Read the model definition and answer for the solid it produces. Units are mm, in the model's axes. Round coordinates to 2 decimals unless told otherwise and drop trailing zeros. Use one line per item in the form item = value. Start each with the question number.
Autodesk Inventor part; units mm, degrees
ref_plane "YZ Plane" through (0, 0, 0) normal (1, 0, 0) x (0, 1, 0)
ref_plane "XZ Plane" through (0, 0, 0) normal (0, 1, 0) x (-1, 0, 0)
ref_plane "XY Plane" through (0, 0, 0) normal (0, 0, 1) x (1, 0, 0)
ref_plane "Work Plane1" through (-113.4922, 95.6302, 200.3599) normal (-0.0001, 0, -1) x (0, -1, 0)
sketch "Sketch1" plane through (-113.4922, 95.6302, 200.3599) normal (-0.0001, 0, -1) x (0, -1, 0)
  line L0 (212.1169, -104.14) -> (330.2269, -104.14)
  line L1 (117.2921, 3.175) -> (320.7139, 3.175)
  line L2 (320.7139, 3.175) -> (320.7139, -104.14)
  line L3 (320.7139, -104.14) -> (117.2921, -104.14)
  line L4 (117.2921, -104.14) -> (117.2921, 3.175)
  circle A0 centre (129.9921, -79.375) radius 2.667
  circle A1 centre (129.9921, -53.975) radius 2.667
  circle A2 centre (129.9921, -28.575) radius 2.667
  circle A3 centre (139.7, -9.525) radius 2.667
  circle A4 centre (165.1, -9.525) radius 2.667
  circle A5 centre (180.3669, -28.575) radius 2.667
  circle A6 centre (180.3669, -53.975) radius 2.667
  circle A7 centre (180.3669, -79.375) radius 2.667
  circle A8 centre (292.1, -9.525) radius 2.667
  circle A9 centre (317.5, -9.525) radius 2.667
  circle A10 centre (266.7, -9.525) radius 2.667
  circle A11 centre (241.3, -9.525) radius 2.667
  circle A12 centre (215.9, -9.525) radius 2.667
  circle A13 centre (190.5, -9.525) radius 2.667
  circle A14 centre (295.3019, -72.39) radius 2.667
  circle A15 centre (269.9019, -72.39) radius 2.667
  circle A16 centre (244.5019, -72.39) radius 2.667
  circle A17 centre (219.1019, -72.39) radius 2.667
  point P0 (95.6298, -113.5035)
extrude "Extrusion1" add sketch "Sketch1" along normal blind 6.35
properties part number "Aluminum Final"
1) Straight lines are drawn through the part: line 1 (Y direction, x = -41, z = 195.25); line 2 (Y direction, x = -33, z = 198.5); line 3 (X direction, y = -32, z = 197). For each, find the intervals that lie inside material, in ascending order. Write a range as from..to.
2) A cutting plane is placed at A-A on z = 198.5. Count the separate pieces of the cut face and the enclosed holes in it, plus the area to 3 significant figures.
3) Determine the mould class of faces 1 (the cylindrical face through (-82.273, -84.39, 197.229)), 2 (the flat face through (-64, -122, 194.01)), 3 (the flat face through (-116.667, -122, 197)) for opening direction X: +X half, -X half, draft (parallel to the pull), parting line (faces both ways), or undercut.
Checks:
q1.line_1 = -225.08..-202.34, -197.01..-176.94, -171.61..-151.54, -146.21..-126.14, -120.81..-21.66
q1.line_2 = -225.08..-87.16, -82.31..-36.78, -31.94..-21.66
q1.line_3 = -116.67..-86.16, -83.68..-60.76, -58.28..-35.36, -32.88..-9.35
q2.separate_pieces = 1
q2.enclosed_holes = 18
q2.area = 21,400 mm²
q3.face_1 = undercut
q3.face_2 = draft
q3.face_3 = -X half
